```python
from build123d import *

# Parameters (mm, degrees)
BOSS_EXTRUDE1_DEPTH     = 25.4
CUT_EXTRUDE1_START      = -6.35
CUT_EXTRUDE1_DEPTH      = 107.95
SKETCH3_W               = 50.8
SKETCH3_H               = 25.4
BOSS_EXTRUDE2_DEPTH     = 6.35
BOSS_EXTRUDE3_START     = -120.65
SKETCH3_2_W             = 50.8
SKETCH3_2_H             = 25.4
BOSS_EXTRUDE3_DEPTH     = 6.35
BOSS_EXTRUDE4_START     = -25.4
SKETCH8_W               = 6.35
SKETCH8_H               = 12.7
BOSS_EXTRUDE4_DEPTH     = 38.1
SKETCH9_R               = 3.2385
CUT_EXTRUDE2_DEPTH      = 1
CUT_EXTRUDE2_DEPTH_BACK = 164.83
SKETCH10_R              = 1.000000032
CUT_EXTRUDE3_DEPTH      = 134.35
SKETCH11_W              = 25.4
SKETCH11_H              = 25.146
BOSS_EXTRUDE5_DEPTH     = 12.7
SKETCH13_W              = 44.45
SKETCH13_H              = 6.35
BOSS_EXTRUDE6_DEPTH     = 12.7
BOSS_EXTRUDE7_START     = -6.35
SKETCH15_W              = 50.8
SKETCH15_H              = 4.826
BOSS_EXTRUDE7_DEPTH     = 19.05
SKETCH17_W              = 50.8
SKETCH17_H              = 0.254
CUT_EXTRUDE4_DEPTH      = 12.7
SKETCH19_W              = 12.7
SKETCH19_H              = 8.763
BOSS_EXTRUDE8_DEPTH     = 113.03
SKETCH20_W              = 106.68
SKETCH20_H              = 0.254
CUT_EXTRUDE5_DEPTH      = 128
SKETCH22_W              = 106.68
SKETCH22_H              = 5.999999938
CUT_EXTRUDE6_DEPTH      = 25.638


with BuildPart() as part:
    # Sketch1 → Boss-Extrude1 (new body)
    with BuildSketch(Plane(origin=(0, 0, 0), x_dir=(1, 0, 0), z_dir=(0, 1, 0))):
        Polygon((3.175, 114.3), (0, 114.3), (0, 120.65), (119.38, 120.65), (119.38, 0), (0, 0), (0, 6.35), (3.175, 6.35), (113.03, 6.35), (113.03, 114.3), align=None)
    extrude(amount=BOSS_EXTRUDE1_DEPTH)

    # Sketch2 → Cut-Extrude1 (cut)
    with BuildSketch(Plane.XY.offset(CUT_EXTRUDE1_START)):
        Polygon((119.38, 25.4), (113.03, 24.13), (113.03, 25.4), align=None)
    extrude(amount=-CUT_EXTRUDE1_DEPTH, mode=Mode.SUBTRACT)

    # Sketch3 → Boss-Extrude2 (add)
    with BuildSketch(Plane.XY):
        with Locations((-19.05, 12.7)):
            Rectangle(SKETCH3_W, SKETCH3_H)
    extrude(amount=BOSS_EXTRUDE2_DEPTH)

    # Sketch3<2> → Boss-Extrude3 (add)
    with BuildSketch(Plane.XY.offset(BOSS_EXTRUDE3_START)):
        with Locations((-19.05, 12.7)):
            Rectangle(SKETCH3_2_W, SKETCH3_2_H)
    extrude(amount=-BOSS_EXTRUDE3_DEPTH)

    # Sketch8 → Boss-Extrude4 (add)
    with BuildSketch(Plane(origin=(0, 25.4, 0), x_dir=(1, 0, 0), z_dir=(0, 1, 0)).offset(BOSS_EXTRUDE4_START)):
        with Locations((116.205, 0)):
            Rectangle(SKETCH8_W, SKETCH8_H)
        with Locations((3.175, 0)):
            Rectangle(SKETCH8_W, SKETCH8_H)
        with Locations((3.175, 120.65)):
            Rectangle(SKETCH8_W, SKETCH8_H)
        with Locations((116.205, 120.65)):
            Rectangle(SKETCH8_W, SKETCH8_H)
    extrude(amount=BOSS_EXTRUDE4_DEPTH)

    # Sketch9 → Cut-Extrude2 (cut, two sides)
    with BuildSketch(Plane(origin=(119.38, 0, 0), x_dir=(0, 0, -1), z_dir=(1, 0, 0))) as cut_extrude2_sk:
        with Locations((0, 31.75)):
            Circle(SKETCH9_R)
        with Locations((120.65, 31.75)):
            Circle(SKETCH9_R)
    extrude(amount=CUT_EXTRUDE2_DEPTH, mode=Mode.SUBTRACT)
    extrude(cut_extrude2_sk.sketch, amount=-CUT_EXTRUDE2_DEPTH_BACK, mode=Mode.SUBTRACT)

    # Sketch10 → Cut-Extrude3 (cut, through all)
    with BuildSketch(Plane.XY.offset(6.35)):
        with Locations((-31.75, 22.225)):
            Circle(SKETCH10_R)
        with Locations((-31.75, 3.175)):
            Circle(SKETCH10_R)
    extrude(amount=-CUT_EXTRUDE3_DEPTH, mode=Mode.SUBTRACT)

    # Sketch11 → Boss-Extrude5 (add)
    with BuildSketch(Plane.XY.offset(6.35)):
        with Locations((-6.35, 12.573)):
            Rectangle(SKETCH11_W, SKETCH11_H)
    extrude(amount=BOSS_EXTRUDE5_DEPTH)

    # Sketch13 → Boss-Extrude6 (add)
    with BuildSketch(Plane(origin=(0, 25.4, 0), x_dir=(1, 0, 0), z_dir=(0, 1, 0))):
        with Locations((-22.225, -3.175)):
            Rectangle(SKETCH13_W, SKETCH13_H)
    extrude(amount=BOSS_EXTRUDE6_DEPTH)

    # Sketch15 → Boss-Extrude7 (add)
    with BuildSketch(Plane.XY.offset(6.35).offset(BOSS_EXTRUDE7_START)):
        with Locations((-19.05, 40.513)):
            Rectangle(SKETCH15_W, SKETCH15_H)
    extrude(amount=BOSS_EXTRUDE7_DEPTH)

    # Sketch17 → Cut-Extrude4 (cut)
    with BuildSketch(Plane.XY.offset(19.05)):
        with Locations((-19.05, 38.227)):
            Rectangle(SKETCH17_W, SKETCH17_H)
    extrude(amount=-CUT_EXTRUDE4_DEPTH, mode=Mode.SUBTRACT)

    # Sketch19 → Boss-Extrude8 (add)
    with BuildSketch(Plane(origin=(6.35, 0, 0), x_dir=(0, 0, -1), z_dir=(1, 0, 0))):
        with Locations((-6.35, 20.2565)):
            Rectangle(SKETCH19_W, SKETCH19_H)
    extrude(amount=BOSS_EXTRUDE8_DEPTH)

    # Sketch20 → Cut-Extrude5 (cut, through all)
    with BuildSketch(Plane.XY):
        with Locations((59.69, 25.273)):
            Rectangle(SKETCH20_W, SKETCH20_H)
    extrude(amount=-CUT_EXTRUDE5_DEPTH, mode=Mode.SUBTRACT)

    # Sketch22 → Cut-Extrude6 (cut, through all)
    with BuildSketch(Plane(origin=(0, 24.638, 0), x_dir=(1, 0, 0), z_dir=(0, 1, 0))):
        with Locations((59.69, -6.35)):
            Rectangle(SKETCH22_W, SKETCH22_H)
    extrude(amount=-CUT_EXTRUDE6_DEPTH, mode=Mode.SUBTRACT)


solid = part.part
```
The listing builds one solid part. Answer for the finished solid, in the listing's coordinates (mm). A direction names the side the tool comes from. Coordinates: 2 decimals unless noted, no trailing zeros. Write each loop counter-clockwise with the first axis right and the second up, starting at its lowest first coordinate (ties: lowest second). Pieces come first, ordered by that corner, then holes. Notation, with made-up numbers: (-7, 45.5) - (41, 45.5) arc R8 cw to (41, 58.5) - close; hole circle Ø8 at (14.5, -28.75). An arc over 180 degrees is marked (long way). Return JSON: item names as keys, results as strings. Group by question number.
1. A cutting plane is placed at D-D, the plane z = -80. Determine the outline of the cut face in (x, y), plus the area to 3 significant figures.
2. Determine the mould class of faces 5 (the flat face through (62, 15.875, 11)), 6 (the flat face through (116, 19, -127)), 7 (the flat face through (0, 19, -3)) for opening direction Z: released by +Z, released by -Z, zero draft, split by the parting line, or undercut.
3. A cutting plane is placed at A-A, the plane x = 48. Determine the outline of the cut face in (y, z) (3 decimals), plus the area to 3 significant figures.
4. Straight lines are drawn through the part: L1, parallel to Y at x = -31.75, z = 1.75 (3 decimals); L2, parallel to Y at x = -31.75, z = -122.75 (3 decimals); L3, parallel to Z at x = 98.5, y = 17.5. For each, find the intervals that lie inside material, in ascending order.
5. A cutting plane is placed at B-B, the plane y = 31.75. Give the number of separate pieces and of enclosed holes in the cut face, plus the area to 3 significant figures.
6. Given pin 1 (7 mm diameter, centred on x = 115, y = 7.5, fed in from +Z); pin 2 (10 mm diameter, centred on y = 8, z = 15, fed in from -X); pin 3 (2 mm diameter, centred on x = 57.5, y = 5, fed in from -Z); pin 4 (6 mm diameter, centred on y = 31.75, z = -120.65, fed in from -X), each flat-ended and moving along its own axis, determine where each tip first touches the part or whether it passes through.
7. Which of the six approach directions +Z, -Z, +X, -X, +Y, -Y give full straight-line access (tool end or side, diameter ignored) to faces 1 (the flat face through (59, 12, -120.65)), 2 (the flat face through (3, 38.1, -121)), 3 (the flat face through (116, 38.1, 0)), 4 (the flat face through (-19.05, 12, 13))?
8. A cutting plane is placed at C-C, the plane y = 9. Determine the outline of the cut face in (x, z).
Ans:
{
 "1": {"outline": "(113.03, 0) - (119.38, 0) - (119.38, 25.4) - (113.03, 24.13) - close", "area": "157 mm²"},
 "2": {"face 5": "zero draft", "face 6": "released by -Z", "face 7": "undercut"},
 "3": {"outline": "(0, -120.65) - (25.146, -120.65) - (25.146, -114.3) - (0, -114.3) - close; (0, -6.35) - (25.146, -6.35) - (25.146, 0) - (24.638, 0) - (24.638, 3.35) - (15.875, 3.35) - (15.875, 0) - (0, 0) - close; (15.875, 9.35) - (24.638, 9.35) - (24.638, 12.7) - (15.875, 12.7) - close", "area": "378 mm²"},
 "4": {"L1": "0 to 2.175, 4.175 to 21.225, 23.225 to 42.926", "L2": "0 to 2.175, 4.175 to 21.225, 23.225 to 25.4", "L3": "-120.65 to -114.3, -6.35 to 3.35, 9.35 to 12.7"},
 "5": {"separate pieces": "8", "enclosed holes": "0", "area": "440 mm²"},
 "6": {"pin 1": "z = 6.35", "pin 2": "x = -19.05", "pin 3": "z = -120.65", "pin 4": "through"},
 "7": {"face 1": "-Z, +Y, -Y", "face 2": "-Z, +X, -X, +Y", "face 3": "+Z, -Z, +X, +Y", "face 4": "+Z, -X, -Y"},
 "8": {"outline": "(-44.45, -127) - (6.35, -127) - (6.35, -120.65) - (113.03, -120.65) - (113.03, -127) - (119.38, -127) - (119.38, 6.35) - (113.03, 6.35) - (113.03, 0) - (6.35, 0) - (6.35, 19.05) - (-19.05, 19.05) - (-19.05, 6.35) - (-44.45, 6.35) - (-44.45, 0) - (0, 0) - (0, -6.35) - (113.03, -6.35) - (113.03, -114.3) - (0, -114.3) - (0, -120.65) - (-44.45, -120.65) - close"}
}
